```python
from build123d import *

# Parameters (mm, degrees)
F0_W     = 50.8
F0_H     = 50.8
F1_DEPTH = 19.05
F2_W     = 6.35
F2_H     = 19.05
F3_DEPTH = 101.601
F4_R     = 3.175
F5_DEPTH = 23.3323898
F6_R     = 3.175
F7_DEPTH = 12.701
F8_R     = 6.35
F9_DEPTH = 6.35
F9_TAPER = 30


with BuildPart() as f1:
    # F0 (on Front) → F1 (new body)
    with BuildSketch(Plane.XZ):
        with Locations((-25.4, 25.4)):
            Rectangle(F0_W, F0_H)
        with Locations((25.4, 25.4)):
            Rectangle(F0_W, F0_H)
    extrude(amount=-F1_DEPTH)

    # F2 (on face) → F3 (cut, through all)
    with BuildSketch(Plane.YZ.offset(50.8)):
        Polygon((0, 50.8), (0, 19.05), (8.5073868597, 50.8), align=None)
        with Locations((3.175, 9.525)):
            Rectangle(F2_W, F2_H)
    extrude(amount=-F3_DEPTH, mode=Mode.SUBTRACT)

    # F4 (on face) → F5 (cut, through all)
    with BuildSketch(Plane(origin=(0, -4.7625, 1.276108029), x_dir=(1, 0, 0), z_dir=(0, -0.9659258263, 0.2588190451))):
        with Locations((0, 37.4508869908)):
            Circle(F4_R)
    extrude(amount=-F5_DEPTH, mode=Mode.SUBTRACT)

    # F6 (on face) → F7 (cut, through all)
    with BuildSketch(Plane.XZ.offset(-6.35)):
        with Locations((0, 9.525)):
            Circle(F6_R)
    extrude(amount=-F7_DEPTH, mode=Mode.SUBTRACT)

    # F8 (on face) → F9 (cut)
    with BuildSketch(Plane.XZ.offset(-6.35)):
        with Locations((0, 9.525)):
            Circle(F8_R)
    extrude(amount=-F9_DEPTH, taper=F9_TAPER, mode=Mode.SUBTRACT)


solid = f1.part
```
Source: CAD feature listing. Evaluate the final solid. Frame: model axes, mm. A direction names the side the tool comes from. Round coordinates to 2 decimals unless told otherwise and drop trailing zeros. Loops run counter-clockwise (first coordinate to the right, second up) from the corner with the lowest first, then second, coordinate; pieces in that order, holes last. Notation, with made-up numbers: M -40,-40 L -25,-40 A17 ccw -25,-9 Z; hole C 80,78.5 d6. An arc over 180 degrees is marked long. Use a Markdown table: item, result. Add a question column.
1. Line query: line 1 (Z direction, x = 0, y = 16); line 2 (Z direction, x = 0, y = 17); line 3 (X direction, y = 11.5, z = 38). Output: solid intervals per line, ascending.
2. Section query A-A on x = 0. Return the cut outline in (y, z) (3 decimals).
3. Mould query, pull axis Y, two halves, no side actions, for faces 1 (the cylindrical face through (-0.688, 11.504, 32.481)), 2 (the flat face through (-1, 19.05, 26)), 3 (the conical face through (3.512, 10.971, 10.631)), 4 (the cylindrical face through (1.71, 15.4, 12.2)). Classes: pulls with the +Y half, pulls with the -Y half, needs draft (parallel to the pull), parting line crosses it, or undercut.
4. Reachability of faces 5 (the flat face through (1, 3, 19.05)), 6 (the flat face through (-50.8, 12, 25)) from +Z, -Z, +X, -X, +Y, -Y: full face, straight path, thin tool, end or side. Return the list, or none.
5. Contact query for flat-ended pins moving along their axis: P1, Ø1.9, axis at x = -13, y = 3, coming from the -Z side; P2, Ø3, axis at x = -3, z = 9.5, coming from the -Y side. Output: stop coordinate, or through.
6. Section query B-B on x = -23.5. Return the cut outline in (y, z).
7. Section query C-C on z = 22.5. Return the cut outline in (x, y).
Reported:
| question | item | result |
|---|---|---|
| 1 | line 1 | z = 0 to 6.35, 12.7 to 31.2, 37.77 to 50.8 |
| 1 | line 2 | z = 0 to 6.35, 12.7 to 30.93, 37.5 to 50.8 |
| 1 | line 3 | x = -50.8 to -2.26, 2.26 to 50.8 |
| 2 | outline | M 0,19.05 L 6.35,19.05 L 6.35,15.875 L 11.849,12.7 L 19.05,12.7 L 19.05,30.381 L 4.109,34.384 Z; M 5.752,40.518 L 19.05,36.955 L 19.05,50.8 L 8.507,50.8 Z; M 6.35,0 L 19.05,0 L 19.05,6.35 L 11.849,6.35 L 6.35,3.175 Z |
| 3 | face 1 | undercut |
| 3 | face 2 | pulls with the +Y half |
| 3 | face 3 | pulls with the -Y half |
| 3 | face 4 | needs draft |
| 4 | face 5 | -Z, +X, -X, -Y |
| 4 | face 6 | +Z, -Z, -X, +Y, -Y |
| 5 | P1 | stops at z = 19.05 |
| 5 | P2 | stops at y = 9.55 |
| 6 | outline | M 0,19.05 L 6.35,19.05 L 6.35,0 L 19.05,0 L 19.05,50.8 L 8.51,50.8 Z |
| 7 | outline | M -50.8,0.92 L 50.8,0.92 L 50.8,19.05 L -50.8,19.05 Z |
